from build123d import *

# Parameters (mm, degrees)
SKETCH_1_W          = 42
SKETCH_1_H          = 42
EXTRUDE_1_DEPTH     = 42
SKETCH_2_R          = 1.5
CUT_EXTRUDE_1_DEPTH = 10
SKETCH_3_R          = 11
EXTRUDE_2_DEPTH     = 1.8
SKETCH_4_R          = 2.5
EXTRUDE_3_DEPTH     = 30


with BuildPart() as part:
    # 草图1 → 凸台-拉伸1 (new body)
    with BuildSketch(Plane.XY):
        Rectangle(SKETCH_1_W, SKETCH_1_H)
    extrude(amount=EXTRUDE_1_DEPTH)

    # 草图2 → 切除-拉伸1 (cut)
    with BuildSketch(Plane.XY.offset(42)):
        with Locations((15.5, 15.5)):
            Circle(SKETCH_2_R)
        with Locations(Location((-15.5, 15.5, 0), (0, 0, 180))):
            Circle(SKETCH_2_R)
        with Locations((-15.5, -15.5)):
            Circle(SKETCH_2_R)
        with Locations(Location((15.5, -15.5, 0), (0, 0, 180))):
            Circle(SKETCH_2_R)
    extrude(amount=-CUT_EXTRUDE_1_DEPTH, mode=Mode.SUBTRACT)

    # 草图3 → 凸台-拉伸2 (add)
    with BuildSketch(Plane.XY.offset(42)):
        Circle(SKETCH_3_R)
    extrude(amount=EXTRUDE_2_DEPTH)

    # 草图4 → 凸台-拉伸3 (add)
    with BuildSketch(Plane.XY.offset(43.8)):
        Circle(SKETCH_4_R)
    extrude(amount=EXTRUDE_3_DEPTH)


solid = part.part
Can you work these out from the model? Positions are in its coordinate system, mm. A direction names the side the tool comes from. Coordinates: 2 decimals unless noted, no trailing zeros. Write each loop counter-clockwise with the first axis right and the second up, starting at its lowest first coordinate (ties: lowest second). Pieces come first, ordered by that corner, then holes. Notation, with made-up numbers: (-1, 22.25) - (11, 22.25) arc R23 ccw to (11, 53.25) - close; hole circle Ø7 at (84, 47.5). An arc over 180 degrees is marked (long way). Return JSON: item names as keys, results as strings. Group by question number.
Item 1: We'd pull the mould along Y, two halves only. Please class faces 3 (the face through (0, 0, 0)), 4 (the face through (16, -16, 32)), 5 (the face through (0, 21, 21)): pulls with the +Y half, pulls with the -Y half, needs draft (parallel to the pull), parting line crosses it, or undercut.
Item 2: If we section it at D-D (y = -8): Write out the boundary of the cut face in (x, z).
Item 3: I'm going to push flat-ended pins straight in: pin 1 Ø2.5 at (x, y) = (15, -15.5) entering from +Z; pin 2 Ø1.5 at (x, z) = (-6, 43) entering from +Y; pin 3 Ø8 at (x, y) = (-1.5, -7) entering from +Z. Where does each tip first touch, or does it pass through?
Item 4: If we section it at A-A (x = 15.5): Write out the boundary of the cut face in (y, z), then the cut area to 3 significant figures.
Item 5: Which directions (+Z, -Z, +X, -X, +Y, -Y) give clear straight access to the entire face, cutting with the end or side of a thin tool? Please do faces 1 (the face through (14, 15.57, 37.07)), 2 (the face through (0, 0, 73.8)).
Item 6: If we section it at C-C (z = 54.5): Write out the boundary of the cut face in (x, y).
Item 7: If we section it at B-B (y = 0): Write out the boundary of the cut face in (x, z), then the cut area to 3 significant figures.
Item 8: Please list where these lines run through material, in increasing order: probe 1 along Y at (x, z) = (-15.5, 35); probe 2 along X at (y, z) = (15, 35).
Return value:
{
 "1": {"face 3": "needs draft", "face 4": "undercut", "face 5": "pulls with the +Y half"},
 "2": {"outline": "(-21, 0) - (21, 0) - (21, 42) - (7.55, 42) - (7.55, 43.8) - (-7.55, 43.8) - (-7.55, 42) - (-21, 42) - close"},
 "3": {"pin 1": "stops at z = 42", "pin 2": "stops at y = 9.67", "pin 3": "stops at z = 43.8"},
 "4": {"outline": "(-21, 0) - (21, 0) - (21, 42) - (17, 42) - (17, 32) - (14, 32) - (14, 42) - (-14, 42) - (-14, 32) - (-17, 32) - (-17, 42) - (-21, 42) - close", "area": "1,700 mm^2"},
 "5": {"face 1": "+Z", "face 2": "+Z, +X, -X, +Y, -Y"},
 "6": {"outline": "circle Ø5 at (0, 0)"},
 "7": {"outline": "(-21, 0) - (21, 0) - (21, 42) - (11, 42) - (11, 43.8) - (2.5, 43.8) - (2.5, 73.8) - (-2.5, 73.8) - (-2.5, 43.8) - (-11, 43.8) - (-11, 42) - (-21, 42) - close", "area": "1,950 mm^2"},
 "8": {"probe 1": "y = -21 to -17, -14 to 14, 17 to 21", "probe 2": "x = -21 to -16.91, -14.09 to 14.09, 16.91 to 21"}
}
